Part model, mm, in its own coordinate system. A direction names the side the tool comes from. Round coordinates to 2 decimals unless told otherwise and drop trailing zeros. Write each loop counter-clockwise with the first axis right and the second up, starting at its lowest first coordinate (ties: lowest second). Pieces come first, ordered by that corner, then holes. Notation, with made-up numbers: (-25.75, 2.25) -> (16.25, 2.25) arc R23 cw to (16.25, 33.25) -> close; hole circle Ø8 at (46.25, 10). An arc over 180 degrees is marked (long way). Return JSON: item names as keys, results as strings. Group by question number.
(1) Mould opens along Y. For faces 1 (the flat face through (-5.483, -9.579, 1.479)), 2 (the flat face through (6.24, 0.53, 1.48)), 3 (the flat face through (30, -63.522, 1)), 4 (the flat face through (-3, -5, 3)) say: +Y half, -Y half, draft (parallel to the pull), parting line (faces both ways), or undercut.
(2) Saw through at B-B (x = 33.5). List the corners of the cut face in (y, z).
(3) Saw through at A-A (y = -9). List the corners of the cut face in (x, z), plus the area to 3 significant figures.
(4) Drop flat-ended pins along their axis: pin 1 Ø1 at (y, z) = (9, 2) entering from +X; pin 2 Ø1 at (y, z) = (-7, 2) entering from -X; pin 3 Ø0.9 at (y, z) = (-62.5, 2) entering from +X. Give the stop position or say it passes through.
(5) Drill centre lines: L1, parallel to Y at x = 5, z = 2.6; L2, parallel to X at y = 55, z = 1.5; L3, parallel to Y at x = 5.5, z = 2.55. Where is each one in solid material? Low to high. Write a range as from..to.
(6) Tool access for faces 5 (the flat face through (-35.057, 46, 1)), 6 (the flat face through (-2, -66.522, 1)), 7 (the flat face through (13, -63.522, 1)), 8 (the flat face through (-3, -5, 0)), 9 (the flat face through (-11.582, -61, 1)): list every direction of +Z, -Z, +X, -X, +Y, -Y with a clear straight run to the whole face (end or side of a thin tool).
from build123d import *

# Parameters (mm, degrees)
F1_DEPTH = 3


# Not quite as in the source:
# - ends of sketch curves that miss each other by under 0.0002 mm in the source are joined


with BuildPart() as f1:
    # F0 (on Top) → F1 (new body)
    with BuildSketch(Plane.XY):
        with BuildLine():
            Line((-11.331514, -63.521951), (-6.04749, -63.521951))
            ThreePointArc((-6.04749, -63.521951), (-5.797538527, -63.4549610061), (-5.6145259066, -63.2719490539))
            ThreePointArc((-5.6145259066, -63.2719490539), (-4.8279591264, -63.1683980924), (-4.9315131291, -63.9549637764))
            ThreePointArc((-4.9315131291, -63.9549637764), (-5.1145256646, -64.1379759355), (-5.181513, -64.387976))
            Line((-5.181513, -64.387976), (-5.181517, -66.022003))
            ThreePointArc((-5.181517, -66.022003), (-5.0350703906, -66.3755563906), (-4.681517, -66.522003))
            Line((-4.681517, -66.522003), (0.318481, -66.522003))
            ThreePointArc((0.318481, -66.522003), (0.6720343906, -66.3755563906), (0.818481, -66.022003))
            Line((0.818481, -66.022003), (0.818481, -64.387974))
            ThreePointArc((0.818481, -64.387974), (0.7514940061, -64.137974527), (0.5684820539, -63.9549619066))
            ThreePointArc((0.5684820539, -63.9549619066), (0.4649300924, -63.1683971264), (1.2514957764, -63.2719511291))
            ThreePointArc((1.2514957764, -63.2719511291), (1.4345099355, -63.4549636646), (1.68451, -63.521951))
            Line((1.68451, -63.521951), (6.818481, -63.521951))
            Line((6.818481, -63.521951), (6.818481, -60.521979))
            Line((6.818481, -60.521979), (5.543485, -60.521979))
            Line((5.543485, -60.521979), (5.543485, -56.521951))
            Line((5.543485, -56.521951), (6.818481, -56.521951))
            Line((6.818481, -56.521951), (6.818481, -53.521951))
            Line((6.818481, -53.521951), (10.018491, -53.521951))
            Line((10.018491, -53.521951), (10.018491, -56.521951))
            Line((10.018491, -56.521951), (11.293485, -56.521951))
            Line((11.293485, -56.521951), (11.293485, -60.521979))
            Line((11.293485, -60.521979), (10.018491, -60.521979))
            Line((10.018491, -60.521979), (10.018491, -63.521951))
            Line((10.018491, -63.521951), (15.152465, -63.521948))
            ThreePointArc((15.152465, -63.521948), (15.4024642565, -63.4549611311), (15.5854768434, -63.2719494869))
            ThreePointArc((15.5854768434, -63.2719494869), (16.3720418736, -63.1683980924), (16.2684878709, -63.9549637764))
            ThreePointArc((16.2684878709, -63.9549637764), (16.0854743354, -64.1379759355), (16.018487, -64.387976))
            Line((16.018487, -64.387976), (16.018484, -66.022003))
            ThreePointArc((16.018484, -66.022003), (16.1649306094, -66.3755563906), (16.518484, -66.522003))
            Line((16.518484, -66.522003), (21.518482, -66.522003))
            ThreePointArc((21.518482, -66.522003), (21.8720353906, -66.3755563906), (22.018482, -66.022003))
            Line((22.018482, -66.022003), (22.018482, -64.387974))
            ThreePointArc((22.018482, -64.387974), (21.9514952226, -64.137974902), (21.7684838039, -63.9549623396))
            ThreePointArc((21.7684838039, -63.9549623396), (21.6649320924, -63.1683971264), (22.4514977764, -63.2719511291))
            ThreePointArc((22.4514977764, -63.2719511291), (22.634510152, -63.4549637896), (22.88451, -63.521951))
            Line((22.88451, -63.521951), (37.957041, -63.521951))
            ThreePointArc((37.957041, -63.521951), (38.0420573761, -63.4746028356), (38.0465663652, -63.3773953159))
            Line((38.0465663652, -63.3773953159), (-26.465295, 66.24561))
            ThreePointArc((-26.465295, 66.24561), (-26.6496426342, 66.4473285217), (-26.912508, 66.522003))
            Line((-26.912508, 66.522003), (-35.056991, 66.522003))
            Line((-35.056991, 66.522003), (-35.056987, 55.98807))
            ThreePointArc((-35.056987, 55.98807), (-34.9900000061, 55.738070527), (-34.8069880539, 55.5550579066))
            ThreePointArc((-34.8069880539, 55.5550579066), (-34.7034372218, 54.768492997), (-35.4900025264, 54.8720466961))
            ThreePointArc((-35.4900025264, 54.8720466961), (-35.6730149355, 55.0550596646), (-35.923015, 55.122047))
            Line((-35.923015, 55.122047), (-37.557041, 55.12205))
            ThreePointArc((-37.557041, 55.12205), (-37.9105943906, 54.9756033906), (-38.057041, 54.62205))
            Line((-38.057041, 54.62205), (-38.057041, 49.622052))
            ThreePointArc((-38.057041, 49.622052), (-37.9105943906, 49.2684986094), (-37.557041, 49.122052))
            Line((-37.557041, 49.122052), (-35.923013, 49.122052))
            ThreePointArc((-35.923013, 49.122052), (-35.673013527, 49.1890389939), (-35.4900009066, 49.3720509461))
            ThreePointArc((-35.4900009066, 49.3720509461), (-34.7034359497, 49.4756017309), (-34.8069901291, 48.6890362236))
            ThreePointArc((-34.8069901291, 48.6890362236), (-34.9900026646, 48.5060240645), (-35.05699, 48.256024))
            Line((-35.05699, 48.256024), (-35.05699, 43.122054))
            Line((-35.05699, 43.122054), (-32.057018, 43.122054))
            Line((-32.057018, 43.122054), (-32.057018, 44.397048))
            Line((-32.057018, 44.397048), (-28.05699, 44.397048))
            Line((-28.05699, 44.397048), (-28.05699, 43.122054))
            Line((-28.05699, 43.122054), (-25.05699, 43.122054))
            Line((-25.05699, 43.122054), (-25.05699, 39.922043))
            Line((-25.05699, 39.922043), (-28.05699, 39.922043))
            Line((-28.05699, 39.922043), (-28.05699, 38.647048))
            Line((-28.05699, 38.647048), (-32.057018, 38.647048))
            Line((-32.057018, 38.647048), (-32.057018, 39.922043))
            Line((-32.057018, 39.922043), (-35.05699, 39.922043))
            Line((-35.05699, 39.922043), (-35.056987, 34.788071))
            ThreePointArc((-35.056987, 34.788071), (-34.9900000061, 34.538071527), (-34.8069880539, 34.3550589066))
            ThreePointArc((-34.8069880539, 34.3550589066), (-34.7034372218, 33.568492997), (-35.4900025264, 33.6720466961))
            ThreePointArc((-35.4900025264, 33.6720466961), (-35.6730149355, 33.8550596646), (-35.923015, 33.922047))
            Line((-35.923015, 33.922047), (-37.557041, 33.92205))
            ThreePointArc((-37.557041, 33.92205), (-37.9105943906, 33.7756033906), (-38.057041, 33.42205))
            Line((-38.057041, 33.42205), (-38.057041, 28.422053))
            ThreePointArc((-38.057041, 28.422053), (-37.9105943906, 28.0684996094), (-37.557041, 27.922053))
            Line((-37.557041, 27.922053), (-35.923013, 27.922053))
            ThreePointArc((-35.923013, 27.922053), (-35.673013527, 27.9890399939), (-35.4900009066, 28.1720519461))
            ThreePointArc((-35.4900009066, 28.1720519461), (-34.7034359497, 28.2756027309), (-34.8069901291, 27.4890372236))
            ThreePointArc((-34.8069901291, 27.4890372236), (-34.9900026646, 27.3060250645), (-35.05699, 27.056025))
            Line((-35.05699, 27.056025), (-35.05699, 21.728049))
            Line((-35.05699, 21.728049), (-34.80699, 21.478049))
            Line((-34.80699, 21.478049), (-25.894542, 21.478049))
            ThreePointArc((-25.894542, 21.478049), (-21.6823966253, 20.2793600017), (-18.7325143305, 17.0425068355))
            Line((-18.7325143305, 17.0425068355), (8.142657, -36.957493))
            ThreePointArc((8.142657, -36.957493), (7.781941119, -44.7340961853), (0.98063, -48.521951))
            Line((0.98063, -48.521951), (-1.581514, -48.521951))
            ThreePointArc((-1.581514, -48.521951), (-8.6525818119, -51.4508831881), (-11.581514, -58.521951))
            Line((-11.581514, -58.521951), (-11.581514, -63.271951))
            Line((-11.581514, -63.271951), (-11.331514, -63.521951))
        make_face()
    extrude(amount=F1_DEPTH)


solid = f1.part
Computed values:
{
 "1": {"face 1": "undercut", "face 2": "+Y half", "face 3": "-Y half", "face 4": "draft"},
 "2": {"outline": "(-63.52, 0) -> (-54.24, 0) -> (-54.24, 3) -> (-63.52, 3) -> close"},
 "3": {"outline": "(-5.77, 0) -> (10.98, 0) -> (10.98, 3) -> (-5.77, 3) -> close", "area": "50.3 mm2"},
 "4": {"pin 1": "x = 2.27", "pin 2": "x = -7.02", "pin 3": "x = 37.83"},
 "5": {"L1": "-63.52..-47.44, -30.64..3.02", "L2": "-37.88..-35.6, -34.57..-20.87", "L3": "-63.52..-47.12, -31.65..2.02"},
 "6": {"face 5": "+Z, -Z, -X", "face 6": "+Z, -Z, +X, -X, -Y", "face 7": "+Z, -Z, -Y", "face 8": "-Z, +X, -X, +Y, -Y", "face 9": "+Z, -Z, -X, -Y"}
}
